For this review, take the finished solid that the model builds, in its own axes (mm). Round coordinates to 2 decimals unless told otherwise and drop trailing zeros. Order: outer loops, then holes, each group sorted by start corner. A loop starts at its lowest first (then second) coordinate and runs counter-clockwise, first axis right, second up. Notation, with made-up numbers: (29, 47.5) - (54, 47.5) arc R10 ccw to (54, 56.5) - close; hole circle Ø11 at (58, 44.5). An arc over 180 degrees is marked (long way). One line per question, with ' | ' between items.
```python
from build123d import *


with BuildPart() as part:
    # Szkic1 → Obrót1 (revolve)
    with BuildSketch(Plane.XY, mode=Mode.PRIVATE) as obr_t1_sk:
        with BuildLine():
            Line((-1.429289322, 5), (1.429289322, 5))
            Line((1.429289322, 5), (1.5, 5.070710678))
            Line((1.5, 5.070710678), (1.5, 5.75))
            Line((1.5, 5.75), (0.6244998, 5.75))
            ThreePointArc((0.6244998, 5.75), (0, 5.45), (-0.6244998, 5.75))
            Line((-0.6244998, 5.75), (-1.5, 5.75))
            Line((-1.5, 5.75), (-1.5, 5.070710678))
            Line((-1.5, 5.070710678), (-1.429289322, 5))
        make_face()
    revolve(obr_t1_sk.sketch.rotate(Axis((-1.5, 0, 0), (1, 0, 0)), 90), axis=Axis((-1.5, 0, 0), (1, 0, 0)))


solid = part.part
```
(1) Mouldability with a two-part tool opening along Z and no side actions: class faces 1 (the cylindrical face through (0, 0, -5)), 2 (the flat face through (1.5, 5, -2)), 3 (the cylindrical face through (1.06, -5.7, -0.75)) as released by +Z, released by -Z, zero draft, split by the parting line, or undercut.
Output values:
face 1: undercut | face 2: zero draft | face 3: split by the parting line
(2) We need section C-C on x = 0.8. State the section outline as (y, z) points.
Output values:
outline: circle Ø11.5 at (0, 0); hole circle Ø10 at (0, 0)
(3) For probe 1 along Z at (x, y) = (-0.95, -0.75); probe 2 along Y at (x, z) = (0.9, -3), list the stretches that pass through material, from the lowest coordinate up. Write a range as [from, to].
Output values:
probe 1: [-5.7, -4.94], [4.94, 5.7] | probe 2: [-4.91, -4], [4, 4.91]
(4) We need section A-A on z = 0. State the section outline as (x, y) points.
Output values:
outline: (-1.5, -5.75) - (-0.62, -5.75) arc R0.8 cw to (0.62, -5.75) - (1.5, -5.75) - (1.5, -5.07) - (1.43, -5) - (-1.43, -5) - (-1.5, -5.07) - close; (-1.5, 5.07) - (-1.43, 5) - (1.43, 5) - (1.5, 5.07) - (1.5, 5.75) - (0.62, 5.75) arc R0.8 cw to (-0.62, 5.75) - (-1.5, 5.75) - close
(5) We need section D-D on x = -0.35. State the section outline as (y, z) points.
Output values:
outline: circle Ø11.06 at (0, 0); hole circle Ø10 at (0, 0)
(6) Insertion check: pin 1 (6 mm diameter, centred on y = -3.5, z = -3, fed in from -X); pin 2 (4 mm diameter, centred on y = 2, z = -0.5, fed in from +X). Each pin has a flat end and moves straight along its axis. Give the tip position at first contact, or say it passes through.
Output values:
pin 1: x = -1.5 | pin 2: through
